```python
from build123d import *

# Parameters (mm, degrees)
CUT_EXTRUDE1_DEPTH = 38.877097962
FILLET1_R          = 1.27


with BuildPart() as part:
    # Sketch1 → Revolve1 (revolve)
    with BuildSketch(Plane.XY, mode=Mode.PRIVATE) as revolve1_sk:
        Polygon((0, 0), (31.75, 0), (31.75, 14.605), (30.226, 14.605), (28.864818102, 9.525), (2.885181898, 9.525), (1.524, 14.605), (0, 14.605), align=None)
    revolve(revolve1_sk.sketch.rotate(Axis((31.75, 0, 0), (1, 0, 0)), 90), axis=Axis((31.75, 0, 0), (1, 0, 0)))

    # Sketch2 → Cut-Extrude1 (cut, through all)
    with BuildSketch(Plane.ZY):
        Polygon((7.478995387, 0), (3.739497694, 6.477), (-3.739497694, 6.477), (-7.478995387, 0), (-3.739497694, -6.477), (3.739497694, -6.477), align=None)
    extrude(amount=-CUT_EXTRUDE1_DEPTH, mode=Mode.SUBTRACT)

    # Fillet1
    fillet1_edges = [part.edges().sort_by_distance(p)[0] for p in [
        (1.524, 0, -14.605),
        (2.885181898, 0, -9.525),
        (28.864818102, 0, -9.525),
        (30.226, 0, -14.605),
    ]]
    fillet(fillet1_edges, radius=FILLET1_R)

    # Sketch3 → Cut-Revolve1 (revolve, cut)
    with BuildSketch(Plane.XY, mode=Mode.PRIVATE) as cut_revolve1_sk:
        Polygon((27.305, -14.605), (25.4, -14.605), (25.4, 14.605), (29.21, 14.605), (29.21, -0.025313637), (27.305, -0.025313637), align=None)
    revolve(cut_revolve1_sk.sketch.rotate(Axis((25.4, 14.605, 0), (0, 1, 0)), 101.039484404), axis=Axis((25.4, 14.605, 0), (0, 1, 0)), mode=Mode.SUBTRACT)


solid = part.part
```
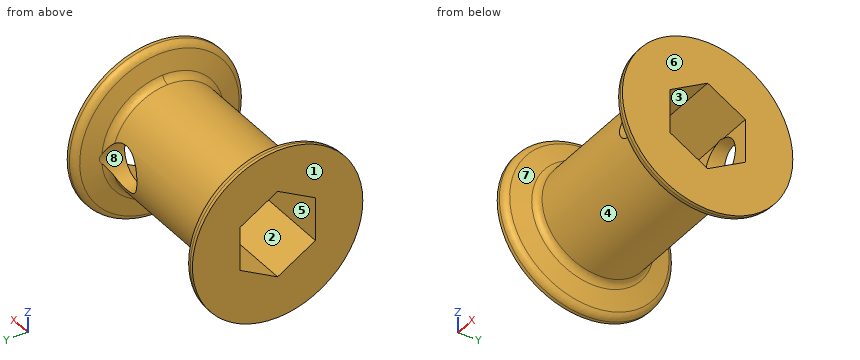
Could you check a few things on this model? Use its own coordinates, in mm. Face numbers are marked on the shaded views. A direction names the side the tool comes from. Round coordinates to 2 decimals unless told otherwise and drop trailing zeros. Answer in a Markdown table with one row per item. Add a question column.
Q1. If I drill on line 1 (X direction, y = -7.7, z = 0) (3 decimals); line 2 (X direction, y = 8.3, z = 0); line 3 (Z direction, x = 23.5, y = 0.75), over which ranges is the centre line in solid material (lowest first)? Write a range as from..to.
Q2. Imagine slicing it at B-B (z = 0). Give the number of separate pieces and of enclosed holes in the cut face, then the cut area to 3 significant figures.
Q3. Will these pins go through, and if not, where does the flat tip stop? pin 1 Ø2 at (x, y) = (5, 11.5) entering from -Z; pin 2 Ø12 at (x, z) = (7.5, -7.5) entering from -Y; pin 3 Ø5 at (x, y) = (8.5, -4.5) entering from -Z; pin 4 Ø8 at (x, z) = (14, 0) entering from +Y (3 decimals).
Q4. On a 3-axis mill with a long thin cutter (end or side, diameter ignored), from which of +Z, -Z, +X, -X, +Y, -Y can I reach the whole of each face in a straight line? I mean the marked faces 5, 6, 7 and 8. Say none if no direction works.
Q5. If we mould it in two halves opening along Y, with no side actions, what happens to the marked faces 1, 2, 3 and 4? For each: +Y half, -Y half, draft (parallel to the pull), parting line (faces both ways), or undercut.
Values:
| question | item | result |
|---|---|---|
| 1 | line 1 | 0..23.495, 27.305..31.75 |
| 1 | line 2 | 0..21.59, 29.21..31.75 |
| 1 | line 3 | -9.5..-7.05, 7.05..9.5 |
| 2 | separate pieces | 4 |
| 2 | enclosed holes | 0 |
| 2 | area | 203 mm^2 |
| 3 | pin 1 | through |
| 3 | pin 2 | y = -12.54 |
| 3 | pin 3 | z = -9.31 |
| 3 | pin 4 | y = 9.525 |
| 4 | face 5 | +X, -X |
| 4 | face 6 | +Z, -Z, +X, +Y, -Y |
| 4 | face 7 | none |
| 4 | face 8 | +Y |
| 5 | face 1 | draft |
| 5 | face 2 | undercut |
| 5 | face 3 | undercut |
| 5 | face 4 | parting line |
